Design review of the part built by this model. Coordinates are the model's own, in mm. A direction names the side the tool comes from. Round coordinates to 2 decimals unless told otherwise and drop trailing zeros. Write each loop counter-clockwise with the first axis right and the second up, starting at its lowest first coordinate (ties: lowest second). Pieces come first, ordered by that corner, then holes. Notation, with made-up numbers: (38, -13.5) -> (93, -13.5) arc R33 cw to (93, 20.5) -> close; hole circle Ø9 at (54.25, 15.5). An arc over 180 degrees is marked (long way). One line per question, with ' | ' between items. Start each with the question number.
1) Consider section D-D (z = -5.5). Give the boundary of the cut face in (x, y), then the cut area to 3 significant figures.
2) For faces 5 (the flat face through (-1, 0, -7.5)), 6 (the flat face through (-1.6, -1.2, 3.4)), list the 3-axis set-ups (+Z, -Z, +X, -X, +Y, -Y) from which the entire face can be reached by the end or side of a thin tool; tool diameter is ignored.
3) For probe 1 along Z at (x, y) = (-1.2, 0); probe 2 along X at (y, z) = (-1, -5.75); probe 3 along Z at (x, y) = (-0.2, -0.5) (3 decimals), list the stretches that pass through material, from the lowest coordinate up.
4) Consider section C-C (y = 0). Give the boundary of the cut face in (x, z), then the cut area to 3 significant figures.
5) Consider section A-A (z = 0). Give the boundary of the cut face in (x, y), then the cut area to 3 significant figures.
6) Mouldability with a two-part tool opening along Y and no side actions: class faces 1 (the cylindrical face through (-1.49, -1.64, -1.26)), 2 (the flat face through (-1, -5, 0)), 3 (the flat face through (-1, 5, 0)), 4 (the flat face through (-3, 2, 2)) as +Y half, -Y half, draft (parallel to the pull), parting line (faces both ways), or undercut.
7) Insertion check: pin 1 Ø1 at (y, z) = (1, -4) entering from -X. The pin has a flat end and moves straight along its axis. Give the tip position at first contact, or say it passes through.
8) Consider section B-B (x = -1.2). Give the boundary of the cut face in (y, z), then the cut area to 3 significant figures.
Autodesk Inventor part; units mm, degrees
ref_plane "dummy_XY" through (0, 0, 0) normal (1, 0, 0) x (0, 0, -1)
ref_plane "dummy_YZ" through (0, 0, 0) normal (0, 0, -1) x (0, 1, 0)
ref_plane "dummy_ZX" through (0, 0, 0) normal (0, 1, 0) x (1, 0, 0)
sketch "Sketch_1" plane through (0, 0, 0) normal (1, 0, 0) x (0, 1, 0)
  line L0 (4.25, 7.5) -> (-4.25, 7.5)
  arc A0 (-4.25, 7.5) -> (-5, 6.75) centre (-4.25, 6.75) ccw
  line L1 (-5, 6.75) -> (-5, -6.75)
  arc A1 (-5, -6.75) -> (-4.25, -7.5) centre (-4.25, -6.75) ccw
  line L2 (-4.25, -7.5) -> (4.25, -7.5)
  arc A2 (4.25, -7.5) -> (5, -6.75) centre (4.25, -6.75) ccw
  line L3 (5, -6.75) -> (5, 6.75)
  arc A3 (5, 6.75) -> (4.25, 7.5) centre (4.25, 6.75) ccw
extrude "Extrusion1" add sketch "Sketch_1" against normal blind 3
sketch "Sketch_2" plane through (0, 0, 0) normal (0, 0, 1) x (1, 0, 0)
  line L0 (3, 0) -> (-3, 0)
  line L1 (-4.6, 3.45) -> (-1.6, 3.45)
  line L2 (-1.6, 3.45) -> (-1.6, 13.45)
  line L3 (-1.6, 13.45) -> (-4.6, 13.45)
  line L4 (-4.6, 13.45) -> (-4.6, 3.45)
revolve "Revolution1" cut sketch "Sketch_2" angle 360 about axis through (3, 0, 0) along (1, 0, 0)
sketch "Sketch_3" plane through (0, 0, 0) normal (0, 0, 1) x (1, 0, 0)
  line L0 (0, 0) -> (-3, 0)
  line L1 (-3, 0) -> (-3, 2.5)
  line L2 (-3, 2.5) -> (-2.567, 2.067)
  line L3 (-2.567, 2.067) -> (-0.433, 2.067)
  line L4 (-0.433, 2.067) -> (0, 2.5)
  line L5 (0, 2.5) -> (0, 0)
  line L6 (0, 0) -> (-3, 0)
revolve "Revolution2" cut sketch "Sketch_3" angle 360 about axis through (0, 0, 0) along (1, 0, 0)
thread "Thread1"
ref_plane "dummy_XY" through (0, 0, 0) normal (1, 0, 0) x (0, 0, -1)
ref_plane "dummy_YZ" through (0, 0, 0) normal (0, 0, -1) x (0, 1, 0)
ref_plane "dummy_ZX" through (0, 0, 0) normal (0, 1, 0) x (1, 0, 0)
properties part number "HNKK5-5"
From the geometry:
1) outline: (-1.6, -5) -> (0, -5) -> (0, 5) -> (-1.6, 5) -> close | area: 16.0 mm2
2) face 5: -Z, +X, -X, +Y, -Y | face 6: -X
3) probe 1: z = -7.5 to -2.07, 2.07 to 7.5 | probe 2: x = -1.6 to 0 | probe 3: z = -7.5 to -2.245, 2.245 to 7.5
4) outline: (-3, -3.45) -> (-1.6, -3.45) -> (-1.6, -7.5) -> (0, -7.5) -> (0, -2.5) -> (-0.43, -2.07) -> (-2.57, -2.07) -> (-3, -2.5) -> close; (-3, 2.5) -> (-2.57, 2.07) -> (-0.43, 2.07) -> (0, 2.5) -> (0, 7.5) -> (-1.6, 7.5) -> (-1.6, 3.45) -> (-3, 3.45) -> close | area: 20.9 mm2
5) outline: (-3, -3.45) -> (-1.6, -3.45) -> (-1.6, -5) -> (0, -5) -> (0, -2.5) -> (-0.43, -2.07) -> (-2.57, -2.07) -> (-3, -2.5) -> close; (-3, 2.5) -> (-2.57, 2.07) -> (-0.43, 2.07) -> (0, 2.5) -> (0, 5) -> (-1.6, 5) -> (-1.6, 3.45) -> (-3, 3.45) -> close | area: 12.9 mm2
6) face 1: undercut | face 2: -Y half | face 3: +Y half | face 4: draft
7) pin 1: stops at x = -1.6
8) outline: (-5, -6.75) arc R0.75 ccw to (-4.25, -7.5) -> (4.25, -7.5) arc R0.75 ccw to (5, -6.75) -> (5, 6.75) arc R0.75 ccw to (4.25, 7.5) -> (-4.25, 7.5) arc R0.75 ccw to (-5, 6.75) -> close; hole circle Ø4.13 at (0, 0) | area: 136 mm2
